Geometry: final body of the model. Coordinates: model frame, mm. Round coordinates to 2 decimals unless told otherwise and drop trailing zeros. Loops run counter-clockwise (first coordinate to the right, second up) from the corner with the lowest first, then second, coordinate; pieces in that order, holes last. Notation, with made-up numbers: (18, 25.5) - (43, 25.5) arc R9 cw to (43, 34.5) - close; hole circle Ø4 at (7, 22). An arc over 180 degrees is marked (long way). Answer as a JSON object with one key per item and string values. Group by question number.
Item 1: Section B-B (y = 2.5). Return the cut outline in (x, z) (3 decimals).
Item 2: First-contact query: pin 1 (1 mm diameter, centred on x = -134, y = 5, fed in from +Z) (3 decimals); pin 2 (2 mm diameter, centred on x = 447, y = -3.5, fed in from +Z) (3 decimals); pin 3 (2 mm diameter, centred on x = 498.5, y = -7, fed in from +Z) (3 decimals). Flat tips, straight axial feed; report the tip coordinate or a pass-through.
Item 3: Line query: line 1 (Y direction, x = 766, z = 25.5) (3 decimals); line 2 (Z direction, x = -393.5, y = -3.5); line 3 (Z direction, x = 649, y = -1.25). Output: solid intervals per line, ascending.
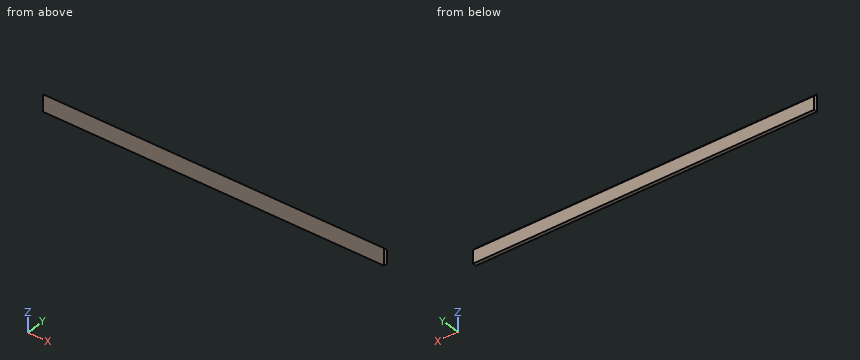
```python
from build123d import *

# Parameters (mm, degrees)
F0_W     = 1801.5966
F0_H     = 88.9
F1_DEPTH = 9.525
F2_SIZE  = 19.04999


# Not quite as in the source:
# - a fillet or chamfer is up to 0.001 mm smaller than in the source, because OpenCascade refuses the exact size


with BuildPart() as f1:
    # F0 (on Front) → F1 (new body, symmetric)
    with BuildSketch(Plane.XZ):
        Rectangle(F0_W, F0_H)
    extrude(amount=F1_DEPTH, both=True)

    # F2 (size 19.05 in the source; OpenCascade refuses exactly that, so slightly less here)
    f2_edges = [f1.edges().sort_by_distance(p)[0] for p in [
        (0, 9.525, 44.45),
    ]]
    chamfer(f2_edges, length=F2_SIZE)


solid = f1.part
```
Values:
{
 "1": {"outline": "(-900.798, -44.45) - (900.798, -44.45) - (900.798, 32.425) - (-900.798, 32.425) - close"},
 "2": {"pin 1": "stops at z = 30.425", "pin 2": "stops at z = 39.425", "pin 3": "stops at z = 42.925"},
 "3": {"line 1": "y = -9.525 to 9.425", "line 2": "z = -44.45 to 38.43", "line 3": "z = -44.45 to 36.18"}
}
